The listing builds one solid part. Answer for the finished solid, in the listing's coordinates (mm). A direction names the side the tool comes from. Coordinates: 2 decimals unless noted, no trailing zeros. Order: outer loops, then holes, each group sorted by start corner. A loop starts at its lowest first (then second) coordinate and runs counter-clockwise, first axis right, second up.
```python
from build123d import *

# Parameters (mm, degrees)
F0_R     = 20.64
F1_DEPTH = 10
F2_R     = 15
F3_DEPTH = 6.3
F4_R     = 11.115
F5_DEPTH = 12.5


with BuildPart() as f1:
    # F0 (on Top) → F1 (new body)
    with BuildSketch(Plane.XY):
        Circle(F0_R)
    extrude(amount=F1_DEPTH)

    # F2 (on Top) → F3 (join, symmetric)
    with BuildSketch(Plane.XY):
        Circle(F2_R)
    extrude(amount=F3_DEPTH, both=True)

    # F4 (on Top) → F5 (cut, symmetric)
    with BuildSketch(Plane.XY):
        Circle(F4_R)
    extrude(amount=F5_DEPTH, both=True, mode=Mode.SUBTRACT)


solid = f1.part
```
(1) Each of these flat-tipped pins is pushed along its axis until it touches: pin 1 Ø2 at (y, z) = (6, -2) entering from -X; pin 2 Ø8 at (x, y) = (-15.5, -12) entering from -Z; pin 3 Ø1.5 at (y, z) = (1.5, -3.5) entering from -X. Where does it stop, or does it pass through?
(2) Consider line 1 (Y direction, x = 0, z = -2.25) (3 decimals); line 2 (Y direction, x = 0, z = 3.75) (3 decimals); line 3 (Z direction, x = 15, y = -3.5). Determine where each line is inside the solid, lowest interval first.
(3) Find section D-D (y = -15.5). Write down the section's boundary in (x, z), and give its area (3 significant figures).
(4) For faces 4 (the face through (-16.38, -12.56, 4.93)), 5 (the face through (-6, -14, 0)), determine the directions among +Z, -Z, +X, -X, +Y, -Y from which every point of the face is accessible in a straight line to the end or side of a thin tool.
(5) The mould has two halves that part along Y. Classify faces 1 (the face through (9, -9, 10)), 2 (the face through (10.6, 3.34, 1.96)), 3 (the face through (-14.985, 0.66, -3.106)): released by +Y, released by -Y, zero draft, split by the parting line, or undercut.
(6) Find section A-A (x = 0). Write down the section's boundary in (y, z) (3 decimals).
(7) Find section C-C (z = 6.75). Write down the section's boundary in (x, y) (3 decimals).
Findings below:
1. pin 1: stops at x = -14.14
1. pin 2: stops at z = 0
1. pin 3: stops at x = -14.98
2. line 1: y = -15 to -11.115, 11.115 to 15
2. line 2: y = -20.64 to -11.115, 11.115 to 20.64
2. line 3: z = 0 to 10
3. outline: (-13.63, 0) - (13.63, 0) - (13.63, 10) - (-13.63, 10) - close
3. area: 273 mm2
4. face 4: +Z, -Z
4. face 5: -Z
5. face 1: zero draft
5. face 2: undercut
5. face 3: split by the parting line
6. outline: (-20.64, 0) - (-15, 0) - (-15, -6.3) - (-11.115, -6.3) - (-11.115, 10) - (-20.64, 10) - close; (11.115, -6.3) - (15, -6.3) - (15, 0) - (20.64, 0) - (20.64, 10) - (11.115, 10) - close
7. outline: circle Ø41.28 at (0, 0); hole circle Ø22.23 at (0, 0)
